from build123d import *

# Parameters (mm, degrees)
F0_W     = 12.7
F0_H     = 38.1
F1_DEPTH = 12.7
F3_D     = 4.4958
F5_D     = 2.4384


with BuildPart() as f1:
    # F0 (on Top) → F1 (new body)
    with BuildSketch(Plane.XY):
        with Locations((6.35, 0)):
            Rectangle(F0_W, F0_H)
    extrude(amount=F1_DEPTH)

    # F3 (through all)
    with Locations(Plane(origin=(0, 0, 0), x_dir=(0, 1, 0), z_dir=(-1, 0, 0))):
        with Locations((0, -6.35)):
            Hole(F3_D / 2)

    # F5 (through all)
    with Locations(Plane(origin=(0, 0, 0), x_dir=(1, 0, 0), z_dir=(0, 0, -1))):
        with Locations((6.35, -10.16), (6.35, 10.16)):
            Hole(F5_D / 2)


solid = f1.part
The listing builds one solid part. Answer for the finished solid, in the listing's coordinates (mm). Coordinates: 2 decimals unless noted, no trailing zeros. Write each loop counter-clockwise with the first axis right and the second up, starting at its lowest first coordinate (ties: lowest second). Pieces come first, ordered by that corner, then holes. Notation, with made-up numbers: (20, 46) - (56, 46) arc R22 cw to (56, 63) - close; hole circle Ø3 at (22.5, 14). An arc over 180 degrees is marked (long way). Put each result on its own line as item: value.
1. The part is cut by section A-A on y = -10.16. Give the vertices of the cut face in (x, z), plus the area to 3 significant figures.
Answer sheet:
outline: (0, 0) - (5.13, 0) - (5.13, 12.7) - (0, 12.7) - close; (7.57, 0) - (12.7, 0) - (12.7, 12.7) - (7.57, 12.7) - close
area: 130 mm^2
2. Find the intervals of material crossed by line 1 along X through (y, z) = (-10.16, 7); line 2 along Z through (x, y) = (6.75, 0); line 3 along Y through (x, z) = (6.35, 7), in increasing order. Write a range as from..to.
Answer sheet:
line 1: x = 0..5.13, 7.57..12.7
line 2: z = 0..4.1, 8.6..12.7
line 3: y = -19.05..-11.38, -8.94..-2.15, 2.15..8.94, 11.38..19.05
3. The part is cut by section B-B on z = 6.35. Give the vertices of the cut face in (x, y), plus the area to 3 significant figures.
Answer sheet:
outline: (0, -19.05) - (12.7, -19.05) - (12.7, -2.25) - (0, -2.25) - close; (0, 2.25) - (12.7, 2.25) - (12.7, 19.05) - (0, 19.05) - close; hole circle Ø2.44 at (6.35, -10.16); hole circle Ø2.44 at (6.35, 10.16)
area: 417 mm^2
4. Determine the mould class of faces 1 (the face through (6.44, 1.78, 7.72)), 2 (the face through (6, 19.05, 6)), 3 (the face through (6, 0, 12.7)) for opening direction Z: pulls with the +Z half, pulls with the -Z half, needs draft (parallel to the pull), parting line crosses it, or undercut.
Answer sheet:
face 1: undercut
face 2: needs draft
face 3: pulls with the +Z half
5. The part is cut by section D-D on z = 9.5. Give the vertices of the cut face in (x, y), plus the area to 3 significant figures.
Answer sheet:
outline: (0, -19.05) - (12.7, -19.05) - (12.7, 19.05) - (0, 19.05) - close; hole circle Ø2.44 at (6.35, -10.16); hole circle Ø2.44 at (6.35, 10.16)
area: 475 mm^2
6. Flat-ended cylindrical pins translate along their axes: pin 1 Ø2 at (x, y) = (6.35, 10.16) entering from -Z; pin 2 Ø1.5 at (x, y) = (8, 10) entering from -Z. Find the tip coordinate at first contact, or state that the pin passes through.
Answer sheet:
pin 1: passes through
pin 2: stops at z = 0
7. The part is cut by section C-C on x = 6.35. Give the vertices of the cut face in (y, z).
Answer sheet:
outline: (-19.05, 0) - (-11.38, 0) - (-11.38, 12.7) - (-19.05, 12.7) - close; (-8.94, 0) - (8.94, 0) - (8.94, 12.7) - (-8.94, 12.7) - close; (11.38, 0) - (19.05, 0) - (19.05, 12.7) - (11.38, 12.7) - close; hole circle Ø4.5 at (0, 6.35)
